from build123d import *

# Parameters (mm, degrees)
F0_W     = 12.7
F0_H     = 12.7
F0_W_2   = 7.62
F0_H_2   = 7.62
F0_W_3   = 6.35
F0_H_3   = 6.35
F1_DEPTH = 12.7
F2_DEPTH = 7.62
F3_DEPTH = 7.62
F4_DEPTH = 5.08
F5_SIZE  = 3.81


with BuildPart() as f1:
    # F0 (on Front) → F1 (new body)
    with BuildSketch(Plane.XZ):
        Rectangle(F0_W, F0_H)
        Rectangle(F0_W_2, F0_H_2, mode=Mode.SUBTRACT)
        Rectangle(F0_W_2, F0_H_2)
        Rectangle(F0_W_3, F0_H_3, mode=Mode.SUBTRACT)
        Rectangle(F0_W_3, F0_H_3)
    extrude(amount=F1_DEPTH)

    # F0 (on Front) → F2 (cut)
    with BuildSketch(Plane.XZ):
        Rectangle(F0_W_3, F0_H_3)
    extrude(amount=F2_DEPTH, mode=Mode.SUBTRACT)

    # F0 (on Front) → F3 (cut)
    with BuildSketch(Plane.XZ):
        Rectangle(F0_W_2, F0_H_2)
        Rectangle(F0_W_3, F0_H_3, mode=Mode.SUBTRACT)
    extrude(amount=F3_DEPTH, mode=Mode.SUBTRACT)

    # F0 (on Front) → F4 (join)
    with BuildSketch(Plane.XZ):
        Rectangle(F0_W_2, F0_H_2)
        Rectangle(F0_W_3, F0_H_3, mode=Mode.SUBTRACT)
    extrude(amount=F4_DEPTH)

    # F5
    f5_edges = [f1.edges().sort_by_distance(p)[0] for p in [
        (-6.35, -6.35, -6.35),
        (6.35, -6.35, -6.35),
        (6.35, -6.35, 6.35),
        (-6.35, -6.35, 6.35),
    ]]
    chamfer(f5_edges, length=F5_SIZE)


solid = f1.part
Part model, mm, in its own coordinate system. A direction names the side the tool comes from. Give positions to 0.01 mm unless a question says otherwise; leave off trailing zeros. Order: outer loops, then holes, each group sorted by start corner. A loop starts at its lowest first (then second) coordinate and runs counter-clockwise, first axis right, second up. Notation, with made-up numbers: (-38.5, 13.5) -> (-30.5, 13.5) arc R19 ccw to (-30.5, 21.5) -> close; hole circle Ø5 at (62.5, 22.5). An arc over 180 degrees is marked (long way). Use one line per item in the form item = value.
(1) Saw through at B-B (x = -2.75). Write the cut outline in (y, z) (3 decimals).
Solution:
outline = (-12.7, -6.14) -> (0, -6.14) -> (0, -3.175) -> (-5.08, -3.175) -> (-5.08, -3.81) -> (-7.62, -3.81) -> (-7.62, 3.81) -> (-5.08, 3.81) -> (-5.08, 3.175) -> (0, 3.175) -> (0, 6.14) -> (-12.7, 6.14) -> close
(2) Saw through at A-A (z = 1.75). Write the cut outline in (x, y) (3 decimals), then the cut area to 3 significant figures.
Solution:
outline = (-6.35, -12.7) -> (6.35, -12.7) -> (6.35, 0) -> (3.175, 0) -> (3.175, -5.08) -> (3.81, -5.08) -> (3.81, -7.62) -> (-3.81, -7.62) -> (-3.81, -5.08) -> (-3.175, -5.08) -> (-3.175, 0) -> (-6.35, 0) -> close
area = 110 mm²
(3) Pull direction Z, two halves, no side cores. Call faces 4 (the face through (0, 0, 4)), 5 (the face through (-3.81, -6, 0)), 6 (the face through (0, -3, -3.175)), 7 (the face through (4.47, -6.26, -4.42)): +Z half, -Z half, draft (parallel to the pull), parting line (faces both ways), or undercut.
Solution:
face_4 = draft
face_5 = undercut
face_6 = undercut
face_7 = -Z half
(4) Saw through at C-C (y = -3.5). Write the cut outline in (x, z) (3 decimals).
Solution:
outline = (-6.35, -2.54) -> (-2.54, -6.35) -> (2.54, -6.35) -> (6.35, -2.54) -> (6.35, 2.54) -> (2.54, 6.35) -> (-2.54, 6.35) -> (-6.35, 2.54) -> close; hole (-3.175, -3.175) -> (3.175, -3.175) -> (3.175, 3.175) -> (-3.175, 3.175) -> close
(5) Saw through at D-D (y = -11.25). Write the cut outline in (x, z), then the cut area to 3 significant figures.
Solution:
outline = (-6.35, -2.54) -> (-2.54, -6.35) -> (2.54, -6.35) -> (6.35, -2.54) -> (6.35, 2.54) -> (2.54, 6.35) -> (-2.54, 6.35) -> (-6.35, 2.54) -> close
area = 132 mm²
(6) Drill centre lines: line 1 (Z direction, x = 2.5, y = -6.5); line 2 (X direction, y = -2.25, z = -1.25) (3 decimals). Where is each one in solid material? Low to high. Write a range as from..to.
Solution:
line_1 = -6.35..-3.81, 3.81..6.35
line_2 = -6.35..-3.175, 3.175..6.35
(7) Tool access for faces 1 (the face through (0, -6, 3.81)), 2 (the face through (0, -6, -6.35)), 3 (the face through (0, -3, 3.175)): list every direction of +Z, -Z, +X, -X, +Y, -Y with a clear straight run to the whole face (end or side of a thin tool).
Solution:
face_1 = none
face_2 = -Z, +X, -X, +Y, -Y
face_3 = +Y
